from build123d import *
from build123d.topology import SkipClean

# Parameters (mm, degrees)
EXTRUDE_1_DEPTH     = 2
SKETCH_2_R          = 2.5
SKETCH_2_R_2        = 1.05
CUT_EXTRUDE_1_DEPTH = 5
SKETCH_4_R          = 1.1
CUT_EXTRUDE_2_DEPTH = 2
EXTRUDE_START       = -2
EXTRUDE_2_DEPTH     = 2
SKETCH_6_OUTSIDE_W  = 57.136
SKETCH_6_OUTSIDE_H  = 39.994
SKETCH_6_OUTSIDE_R  = 12.5
CUT_EXTRUDE_3_DEPTH = 10
EXTRUDE_3_DEPTH     = 2
SKETCH_8_R          = 1.2
CUT_EXTRUDE_4_DEPTH = 10
SKETCH_9_OUTSIDE_W  = 38.188
SKETCH_9_OUTSIDE_H  = 63.188
CUT_EXTRUDE_5_DEPTH = 14
CUT_EXTRUDE_6_DEPTH = 10
SKETCH_11_W         = 2
SKETCH_11_H         = 43.30127019
EXTRUDE_4_DEPTH     = 1.4
EXTRUDE_1_2_DEPTH   = 15


with BuildPart() as part:
    # 草图1 → Extrude 1 (new body)
    with BuildSketch(Plane.XY):
        with BuildLine():
            ThreePointArc((21.650635095, 12.5), (0, 25), (-21.650635095, 12.5))
            ThreePointArc((-21.650635095, 12.5), (-19.820508076, 5.669872981), (-12.990381057, 7.5))
            ThreePointArc((-12.990381057, 7.5), (0, 15), (12.990381057, 7.5))
            ThreePointArc((12.990381057, 7.5), (19.820508076, 5.669872981), (21.650635095, 12.5))
        make_face()
    extrude(amount=EXTRUDE_1_DEPTH)

    # 草图2 → 切除-拉伸1 (cut)
    with BuildSketch(Plane.XY.offset(2)):
        with Locations((0, 20)):
            Circle(SKETCH_2_R)
        with Locations((-5.5, 20)):
            Circle(SKETCH_2_R_2)
        with Locations((5.5, 20)):
            Circle(SKETCH_2_R_2)
    extrude(amount=-CUT_EXTRUDE_1_DEPTH, mode=Mode.SUBTRACT)

    # 草图4 → 切除-拉伸2 (cut)
    with BuildSketch(Plane.XY.offset(2)):
        with Locations((-17.320508076, 10)):
            Circle(SKETCH_4_R)
        with Locations((17.320508076, 10)):
            Circle(SKETCH_4_R)
    extrude(amount=-CUT_EXTRUDE_2_DEPTH, mode=Mode.SUBTRACT)

    # 草图5 → 凸台-拉伸2 (add)
    with BuildSketch(Plane.XY.offset(2).offset(EXTRUDE_START)):
        with BuildLine():
            ThreePointArc((-9.363273917, 11.71875), (0, 7.5), (9.363273917, 11.71875))
            ThreePointArc((9.363273917, 11.71875), (0, 15), (-9.363273917, 11.71875))
        make_face()
        with BuildLine():
            ThreePointArc((12.381272085, 21.71875), (0, 25), (-12.381272085, 21.71875))
            ThreePointArc((-12.381272085, 21.71875), (0, 32.5), (12.381272085, 21.71875))
        make_face()
    extrude(amount=EXTRUDE_2_DEPTH)

    # 草图6 outside → 切除-拉伸3 (cut)
    with SkipClean():  # the faces are left unmerged after this step: merging them gives an invalid solid
        with BuildSketch(Plane.XY.offset(2)):
            with Locations((0, 18.75)):
                Rectangle(SKETCH_6_OUTSIDE_W, SKETCH_6_OUTSIDE_H)
            with Locations((0, 20)):
                Circle(SKETCH_6_OUTSIDE_R, mode=Mode.SUBTRACT)
        extrude(amount=-CUT_EXTRUDE_3_DEPTH, mode=Mode.SUBTRACT)

    # 草图7 → 凸台-拉伸3 (add)
    with SkipClean():  # the faces are left unmerged after this step: merging them gives an invalid solid
        with BuildSketch(Plane.XY.offset(2)):
            with BuildLine():
                Line((-7.5, 10), (-7.5, -5))
                Line((-7.5, -5), (7.5, -5))
                Line((7.5, -5), (7.5, 10))
                ThreePointArc((7.5, 10), (0, 7.5), (-7.5, 10))
            make_face()
            with BuildLine():
                Line((-7.5, 45), (7.5, 45))
                Line((7.5, 45), (7.5, 30))
                ThreePointArc((7.5, 30), (0, 32.5), (-7.5, 30))
                Line((-7.5, 30), (-7.5, 45))
            make_face()
        extrude(amount=-EXTRUDE_3_DEPTH)

    # 草图8 → 切除-拉伸4 (cut)
    with SkipClean():  # the faces are left unmerged after this step: merging them gives an invalid solid
        with BuildSketch(Plane.XY.offset(2)):
            with Locations((-3, 4)):
                Circle(SKETCH_8_R)
            with Locations((-3, 36)):
                Circle(SKETCH_8_R)
        extrude(amount=-CUT_EXTRUDE_4_DEPTH, mode=Mode.SUBTRACT)

    # 草图9 outside → 切除-拉伸5 (cut)
    with SkipClean():  # the faces are left unmerged after this step: merging them gives an invalid solid
        with BuildSketch(Plane.XY.offset(2)):
            with Locations((0, 20)):
                Rectangle(SKETCH_9_OUTSIDE_W, SKETCH_9_OUTSIDE_H)
            with BuildLine():
                ThreePointArc((4.427083333, 8.310220996), (12.5, 20), (4.427083333, 31.689779004))
                ThreePointArc((4.427083333, 31.689779004), (1.965433704, 33.044090503), (-0.022321429, 35.029715862))
                ThreePointArc((-0.022321429, 35.029715862), (-0.269391354, 35.352624611), (-0.52168006, 35.671472564))
                ThreePointArc((-0.52168006, 35.671472564), (-1.179500018, 37.713411748), (-3.177861224, 38.493665051))
                ThreePointArc((-3.177861224, 38.493665051), (-45, 20), (-3.177861224, 1.506334949))
                ThreePointArc((-3.177861224, 1.506334949), (-1.179500018, 2.286588252), (-0.52168006, 4.328527436))
                ThreePointArc((-0.52168006, 4.328527436), (-0.269391354, 4.647375389), (-0.022321429, 4.970284138))
                ThreePointArc((-0.022321429, 4.970284138), (1.965433704, 6.955909497), (4.427083333, 8.310220996))
            make_face(mode=Mode.SUBTRACT)
        extrude(amount=-CUT_EXTRUDE_5_DEPTH, mode=Mode.SUBTRACT)

    # 草图10 → 切除-拉伸6 (cut)
    with SkipClean():  # the faces are left unmerged after this step: merging them gives an invalid solid
        with BuildSketch(Plane(origin=(0, 0, 0), x_dir=(-1, 0, 0), z_dir=(0, 0, -1))):
            Polygon((7.5, 35.825317547), (7.5, 4.174682453), (36.824100737, 12.604038964), align=None)
        extrude(amount=-CUT_EXTRUDE_6_DEPTH, mode=Mode.SUBTRACT)

    # 草图11 → 凸台-拉伸4 (add)
    with SkipClean():  # the faces are left unmerged after this step: merging them gives an invalid solid
        with BuildSketch(Plane.ZY.offset(7.5)):
            with Locations((1, 20)):
                Rectangle(SKETCH_11_W, SKETCH_11_H)
        extrude(amount=EXTRUDE_4_DEPTH)

    # 草图12 → Extrude 1 2 (add)
    with SkipClean():  # the faces are left unmerged after this step: merging them gives an invalid solid
        with BuildSketch(Plane(origin=(0, 0, 0), x_dir=(-1, 0, 0), z_dir=(0, 0, -1))):
            with BuildLine():
                Line((8.9, 7.5), (0, 7.5))
                ThreePointArc((0, 7.5), (-12.5, 20), (0, 32.5))
                Line((0, 32.5), (8.9, 32.5))
                Line((8.9, 32.5), (8.9, 31.5))
                Line((8.9, 31.5), (0, 31.5))
                ThreePointArc((0, 31.5), (-11.5, 20), (0, 8.5))
                Line((0, 8.5), (8.9, 8.5))
                Line((8.9, 8.5), (8.9, 7.5))
            make_face()
        extrude(amount=EXTRUDE_1_2_DEPTH)


solid = part.part
Could you check a few things on this model? Use its own coordinates, in mm. A direction names the side the tool comes from. Give positions to 0.01 mm unless a question says otherwise; leave off trailing zeros. Order: outer loops, then holes, each group sorted by start corner. A loop starts at its lowest first (then second) coordinate and runs counter-clockwise, first axis right, second up.
1. Suppose I cut it at A-A (x = 0.5). Write out the boundary of the cut face in (y, z).
Answers below:
outline: (5.61, 0) - (7.51, 0) - (7.51, -15) - (8.51, -15) - (8.51, 0) - (17.55, 0) - (17.55, 2) - (5.61, 2) - close; (22.45, 0) - (31.49, 0) - (31.49, -15) - (32.49, -15) - (32.49, 0) - (34.39, 0) - (34.39, 2) - (22.45, 2) - close
2. Which directions (+Z, -Z, +X, -X, +Y, -Y) give clear straight access to the entire face, cutting with the end or side of a thin tool? Please do faces 5 (the flat face through (-8, -1.651, 1)), 6 (the flat face through (-4, 8.5, -7)).
Answers below:
face 5: +Z, -Z, +X, -X, -Y
face 6: -Z, -X
3. Suppose I cut it at B-B (z = -5.5). Write out the boundary of the cut face in (x, y).
Answers below:
outline: (-8.9, 7.5) - (0, 7.5) arc R12.5 ccw to (0, 32.5) - (-8.9, 32.5) - (-8.9, 31.5) - (0, 31.5) arc R11.5 cw to (0, 8.5) - (-8.9, 8.5) - close
4. Suppose I cut it at D-D (x = 8.75). Write out the boundary of the cut face in (y, z).
Answers below:
outline: (11.07, -15) - (12.54, -15) - (12.54, 0) - (27.46, 0) - (27.46, -15) - (28.93, -15) - (28.93, 2) - (11.07, 2) - close
5. Suppose I cut it at C-C (y = 23). Write out the boundary of the cut face in (x, z), plus the area to 3 significant figures.
Answers below:
outline: (-8.9, 0) - (11.1, 0) - (11.1, -15) - (12.13, -15) - (12.13, 2) - (-8.9, 2) - close
area: 57.6 mm2
6. I need wall thicknesses on L1, parallel to Y at x = -3, z = 0.6; L2, parallel to Y at x = -5, z = -10; L3, parallel to Z at x = 6, y = 17. Which ranges of each line are inside material? Lowest first, please.
Answers below:
L1: y = 1.5 to 2.8, 5.2 to 34.8, 37.2 to 38.5
L2: y = 7.5 to 8.5, 31.5 to 32.5
L3: z = 0 to 2
7. Thinking about a two-plate mould opening in X: for faces 1 (the cylindrical face through (1.93, 6.93, 1.01)), 2 (the cylindrical face through (5.272, 18.975, 1.014)), 3 (the flat face through (-5, 7.5, -7)), 4 (the cylindrical face through (-0.33, 22.48, 1.01)), which applies, +X half, -X half, draft (parallel to the pull), parting line (faces both ways), or undercut?
Answers below:
face 1: +X half
face 2: undercut
face 3: draft
face 4: undercut
8. For pin 1 (2.5 mm diameter, centred on x = 5.5, y = 20, fed in from -Z); pin 2 (8 mm diameter, centred on x = 5, z = -2.5, fed in from -Y); pin 3 (10 mm diameter, centred on y = 18, z = -11.5, fed in from -X); pin 4 (1.4 mm diameter, centred on x = -3, y = 36, fed in from -Z), each with a flat end and sliding along its axis, tell me the tip position at first contact or that it passes through.
Answers below:
pin 1: stops at z = 0
pin 2: stops at y = 6.89
pin 3: stops at x = 9.12
pin 4: passes through
